from build123d import *

# Parameters (mm, degrees)
Y_KSEKLIK_EKSTR_ZYON1_DEPTH = 30
IZIM2_R                     = 1.5
IZIM2_R_2                   = 3.5
KES_EKSTR_ZYON1_DEPTH       = 58.662812973


with BuildPart() as part:
    # Çizim1 → Yükseklik-Ekstrüzyon1 (new body)
    with BuildSketch(Plane(origin=(0, 0, 0), x_dir=(1, 0, 0), z_dir=(0, 1, 0))):
        with BuildLine():
            Line((20, 40), (20, 34.641016151))
            ThreePointArc((20, 34.641016151), (0, 40), (-20, 34.641016151))
            Line((-20, 34.641016151), (-20, 45))
            Line((-20, 45), (20, 45))
            Line((20, 45), (20, 40))
        make_face()
    extrude(amount=Y_KSEKLIK_EKSTR_ZYON1_DEPTH)

    # Çizim2 → Kes-Ekstrüzyon1 (cut, through all)
    with BuildSketch(Plane.XY):
        with Locations((-5, 5)):
            Circle(IZIM2_R)
        with Locations((5, 5)):
            Circle(IZIM2_R)
        with Locations((5, 25)):
            Circle(IZIM2_R)
        with Locations((-5, 25)):
            Circle(IZIM2_R)
        with Locations((0, 15)):
            Circle(IZIM2_R_2)
    extrude(amount=-KES_EKSTR_ZYON1_DEPTH, mode=Mode.SUBTRACT)


solid = part.part
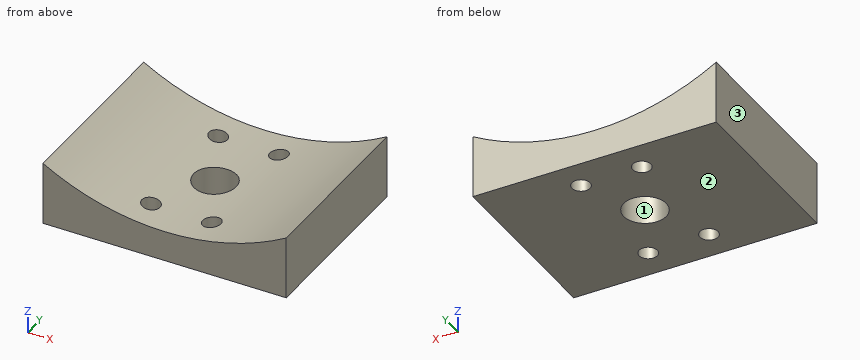
CAD build for the part. Positions are in the model's coordinates, mm. Face numbers are marked on the shaded views. Give positions to 0.01 mm unless a question says otherwise; leave off trailing zeros. Loops run counter-clockwise (first coordinate to the right, second up) from the corner with the lowest first, then second, coordinate; pieces in that order, holes last. Notation, with made-up numbers: M -25.5,68 L -5.5,68 A17 ccw -5.5,73 Z; hole C 82,25.5 d3. An arc over 180 degrees is marked long. One line per question, with ' | ' between items. Start each with the question number.
1. Saw through at C-C on x = 0. Give the cut face in (y, z), plus the area to 3 significant figures.
2. Flat gauge pins, fed straight in: pin 1 (6 mm diameter, centred on x = -4, z = -38.5, fed in from -Y); pin 2 (5 mm diameter, centred on x = -5, y = 25, fed in from +Z); pin 3 (8 mm diameter, centred on x = 5, y = 19.5, fed in from +Z); pin 4 (12 mm diameter, centred on x = 9, y = 16.5, fed in from +Z). Where does each tip first touch, or does it go through?
3. Saw through at D-D on z = -43.5. Give the cut face in (x, y), plus the area to 3 significant figures.
4. Probe L1, parallel to X at y = 25, z = -44.5; L2, parallel to Y at x = 0, z = -42.15; L3, parallel to X at y = 15, z = -43.85. List the from-to ranges inside material, lowest first. Write a range as from..to.
5. Saw through at B-B on y = 5. Give the cut face in (x, z), plus the area to 3 significant figures.
6. Saw through at A-A on y = 15. Give the cut face in (x, z).
7. Two-plate mould, pull along X, no slides. Class the marked faces 1, 2 and 3: pulls with the +X half, pulls with the -X half, needs draft (parallel to the pull), parting line crosses it, or undercut.
Result sheet:
1) outline: M 0,-45 L 11.5,-45 L 11.5,-40 L 0,-40 Z; M 18.5,-45 L 30,-45 L 30,-40 L 18.5,-40 Z | area: 115 mm^2
2) pin 1: stops at y = 0 | pin 2: stops at z = -39.29 | pin 3: stops at z = -38.97 | pin 4: stops at z = -37.08
3) outline: M -20,0 L 20,0 L 20,30 L -20,30 Z; hole C -5,5 d3; hole C -5,25 d3; hole C 0,15 d7; hole C 5,5 d3; hole C 5,25 d3 | area: 1,130 mm^2
4) L1: x = -20..-6.5, -3.5..3.5, 6.5..20 | L2: y = 0..11.5, 18.5..30 | L3: x = -20..-3.5, 3.5..20
5) outline: M -20,-45 L -6.5,-45 L -6.5,-39.47 A40 cw -20,-34.64 Z; M -3.5,-45 L 3.5,-45 L 3.5,-39.85 A40 cw -3.5,-39.85 Z; M 6.5,-45 L 20,-45 L 20,-34.64 A40 cw 6.5,-39.47 Z | area: 237 mm^2
6) outline: M -20,-45 L -3.5,-45 L -3.5,-39.85 A40 cw -20,-34.64 Z; M 3.5,-45 L 20,-45 L 20,-34.64 A40 cw 3.5,-39.85 Z
7) face 1: undercut | face 2: needs draft | face 3: pulls with the -X half
